Geometry: final body of the model. Coordinates: model frame, mm. Face numbers are marked on the shaded views. A direction names the side the tool comes from. Give positions to 0.01 mm unless a question says otherwise; leave off trailing zeros. Write each loop counter-clockwise with the first axis right and the second up, starting at its lowest first coordinate (ties: lowest second). Pieces come first, ordered by that corner, then holes. Notation, with made-up numbers: (14, 28) -> (19, 28) arc R24 cw to (19, 46) -> close; hole circle Ø3 at (75, 1.25). An arc over 180 degrees is marked (long way). Answer in a Markdown table with one row per item. Add a question column.
Item 1: Section query B-B on x = -5. Output: boundary loops of the cut face in (y, z), plus the area to 3 significant figures.
Item 2: First-contact query: P1, Ø1.6, axis at y = 1, z = -1, coming from the +X side; P2, Ø2, axis at x = 2, z = -4.5, coming from the +Y side; P3, Ø1, axis at y = 1, z = 5.5, coming from the -X side. Flat tips, straight axial feed; report the tip coordinate or a pass-through.
Item 3: Material intervals for probe 1 along Z at (x, y) = (9.75, 2.3); probe 2 along X at (y, z) = (1.7, -2.5); probe 3 along Y at (x, z) = (0.5, 10.5), sorted ascending. Write a range as from..to.
Item 4: Access query for the marked faces 1 and 2. Directions: +Z, -Z, +X, -X, +Y, -Y. A direction counts if a zero-diameter tool reaches every point of the face in a straight line with its end or side. Return the directions, or none.
Item 5: Section query D-D on x = -0.5. Output: boundary loops of the cut face in (y, z).
Item 6: Section query C-C on y = 0.55. Output: boundary loops of the cut face in (x, z), plus the area to 3 significant figures.
Item 7: Section query A-A on y = 3.6. Output: boundary loops of the cut face in (x, z), plus the area to 3 significant figures.
Item 8: Draft query along Z for the marked faces 3, 4 and 5. Return one class per face: +Z half, -Z half, draft (parallel to the pull), parting line (faces both ways), or undercut.
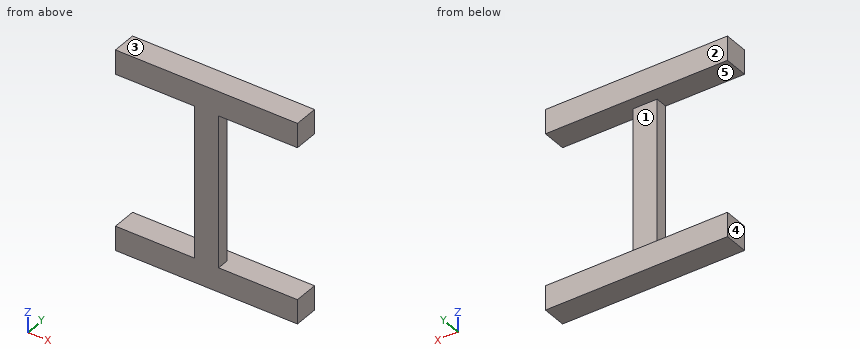
```python
from build123d import *

# Parameters (mm, degrees)
BOSS_EXTRUDE1_DEPTH = 4
SKETCH2_W           = 4
SKETCH2_H           = 25
CUT_EXTRUDE1_DEPTH  = 2


with BuildPart() as part:
    # Sketch1 → Boss-Extrude1 (new body)
    with BuildSketch(Plane(origin=(0, 0, 0), x_dir=(1, 0, 0), z_dir=(0, 1, 0))):
        Polygon((-15, 12.5), (-2, 12.5), (-2, -12.5), (-15, -12.5), (-15, -16.5), (15, -16.5), (15, -12.5), (2, -12.5), (2, 12.5), (15, 12.5), (15, 16.5), (-15, 16.5), align=None)
    extrude(amount=BOSS_EXTRUDE1_DEPTH)

    # Sketch2 → Cut-Extrude1 (cut)
    with BuildSketch(Plane(origin=(0, 4, 0), x_dir=(1, 0, 0), z_dir=(0, 1, 0))):
        Rectangle(SKETCH2_W, SKETCH2_H)
    extrude(amount=-CUT_EXTRUDE1_DEPTH, mode=Mode.SUBTRACT)


solid = part.part
```
Findings below:
| question | item | result |
|---|---|---|
| 1 | outline | (0, -16.5) -> (4, -16.5) -> (4, -12.5) -> (0, -12.5) -> close; (0, 12.5) -> (4, 12.5) -> (4, 16.5) -> (0, 16.5) -> close |
| 1 | area | 32.0 mm^2 |
| 2 | P1 | stops at x = 2 |
| 2 | P2 | stops at y = 2 |
| 2 | P3 | stops at x = -2 |
| 3 | probe 1 | z = -16.5..-12.5, 12.5..16.5 |
| 3 | probe 2 | x = -2..2 |
| 3 | probe 3 | y = 0..2 |
| 4 | face 1 | +X, -X, +Y |
| 4 | face 2 | +Z, -Z, +X, -X, +Y |
| 5 | outline | (0, -16.5) -> (4, -16.5) -> (4, -12.5) -> (2, -12.5) -> (2, 12.5) -> (4, 12.5) -> (4, 16.5) -> (0, 16.5) -> close |
| 6 | outline | (-15, -16.5) -> (15, -16.5) -> (15, -12.5) -> (2, -12.5) -> (2, 12.5) -> (15, 12.5) -> (15, 16.5) -> (-15, 16.5) -> (-15, 12.5) -> (-2, 12.5) -> (-2, -12.5) -> (-15, -12.5) -> close |
| 6 | area | 340 mm^2 |
| 7 | outline | (-15, -16.5) -> (15, -16.5) -> (15, -12.5) -> (-15, -12.5) -> close; (-15, 12.5) -> (15, 12.5) -> (15, 16.5) -> (-15, 16.5) -> close |
| 7 | area | 240 mm^2 |
| 8 | face 3 | +Z half |
| 8 | face 4 | draft |
| 8 | face 5 | undercut |
